Can you work these out from the model? Positions are in its coordinate system, mm. Round coordinates to 2 decimals unless told otherwise and drop trailing zeros. Order: outer loops, then holes, each group sorted by start corner. A loop starts at its lowest first (then second) coordinate and runs counter-clockwise, first axis right, second up.
Q1. If I drill on line 1 (X direction, y = -0.8, z = 7); line 2 (Z direction, x = -76, y = -0.2), over which ranges is the centre line in solid material (lowest first)?
Q2. Will these pins go through, and if not, where does the flat tip stop? P1, Ø1.9, axis at x = 15.5, y = -2, coming from the +Z side; P2, Ø1.1, axis at y = -1.5, z = 25, coming from the +X side; P3, Ø1.1, axis at y = -1.5, z = 25.5, coming from the -X side.
Q3. If we section it at B-B (y = -2.7): Please give me the cut outline in (x, z).
Q4. If we section it at A-A (z = 16): Please give me the cut outline in (x, y), plus the area to 3 significant figures.
Q5. If we section it at C-C (x = -0.5): Please give me the cut outline in (y, z).
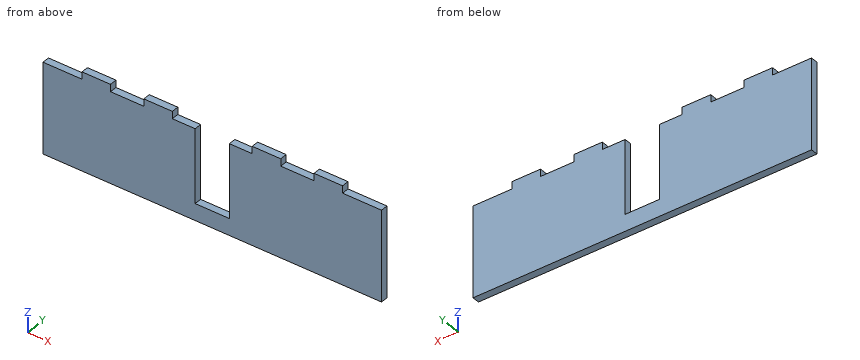
from build123d import *

# Parameters (mm, degrees)
F0_W     = 15
F0_H     = 3.81
F1_DEPTH = 3.81


with BuildPart() as f1:
    # F0 (on Front) → F1 (new body)
    with BuildSketch(Plane.XZ):
        Polygon((89, -23.79), (89, 23.79), (68.5, 23.79), (53.5, 23.79), (36, 23.79), (21, 23.79), (9, 23.79), (9, 0), (9, -15), (0, -15), (0, -23.79), align=None)
        Polygon((-89, -23.79), (0, -23.79), (0, -15), (-9, -15), (-9, 0), (-9, 23.79), (-21, 23.79), (-36, 23.79), (-53.5, 23.79), (-68.5, 23.79), (-89, 23.79), align=None)
        with Locations((-61, 25.695)):
            Rectangle(F0_W, F0_H)
        with Locations((-28.5, 25.695)):
            Rectangle(F0_W, F0_H)
        with Locations((28.5, 25.695)):
            Rectangle(F0_W, F0_H)
        with Locations((61, 25.695)):
            Rectangle(F0_W, F0_H)
    extrude(amount=F1_DEPTH)


solid = f1.part
Solution:
1. line 1: x = -89 to -9, 9 to 89
1. line 2: z = -23.79 to 23.79
2. P1: stops at z = 23.79
2. P2: stops at x = 68.5
2. P3: stops at x = -68.5
3. outline: (-89, -23.79) - (89, -23.79) - (89, 23.79) - (68.5, 23.79) - (68.5, 27.6) - (53.5, 27.6) - (53.5, 23.79) - (36, 23.79) - (36, 27.6) - (21, 27.6) - (21, 23.79) - (9, 23.79) - (9, -15) - (-9, -15) - (-9, 23.79) - (-21, 23.79) - (-21, 27.6) - (-36, 27.6) - (-36, 23.79) - (-53.5, 23.79) - (-53.5, 27.6) - (-68.5, 27.6) - (-68.5, 23.79) - (-89, 23.79) - close
4. outline: (-89, -3.81) - (-9, -3.81) - (-9, 0) - (-89, 0) - close; (9, -3.81) - (89, -3.81) - (89, 0) - (9, 0) - close
4. area: 610 mm2
5. outline: (-3.81, -23.79) - (0, -23.79) - (0, -15) - (-3.81, -15) - close
